```python
from build123d import *

# Parameters (mm, degrees)
SKETCH2_W          = 3.5
SKETCH2_H          = 3.5
CUT_EXTRUDE1_DEPTH = 8.1086


with BuildPart() as part:
    # Sketch1 → Revolve1 (revolve)
    with BuildSketch(Plane.XY):
        Polygon((1.957910998, 0), (0, 0), (0, -2.01497422), (0, -7.1086), (3.0734, -7.1086), (3.0734, -3), (60, -3), (60, 0), align=None)
    revolve(axis=Axis((0, 0, 0), (0, -1, 0)))

    # Sketch2 → Cut-Extrude1 (cut, through all)
    with BuildSketch(Plane(origin=(0, 0, 0), x_dir=(1, 0, 0), z_dir=(0, 1, 0))):
        with BuildLine():
            Line((2.37773001, -1.17), (-2.37773001, -1.17))
            ThreePointArc((-2.37773001, -1.17), (0, 2.65), (2.37773001, -1.17))
        make_face()
        with Locations((-42.92, 0)):
            Rectangle(SKETCH2_W, SKETCH2_H)
        with Locations((0, -42.92)):
            Rectangle(SKETCH2_W, SKETCH2_H)
        with Locations((0, 42.92)):
            Rectangle(SKETCH2_W, SKETCH2_H)
        with Locations((42.92, 0)):
            Rectangle(SKETCH2_W, SKETCH2_H)
    extrude(amount=-CUT_EXTRUDE1_DEPTH, mode=Mode.SUBTRACT)


solid = part.part
```
Verification items for the finished model (mm, model axes). A direction names the side the tool comes from. Give positions to 0.01 mm unless a question says otherwise; leave off trailing zeros. Order: outer loops, then holes, each group sorted by start corner. A loop starts at its lowest first (then second) coordinate and runs counter-clockwise, first axis right, second up. Notation, with made-up numbers: M 17,-6.5 L 52,-6.5 A15 cw 52,10.5 Z; hole C 11.5,26.5 d6. An arc over 180 degrees is marked long. Return JSON: item names as keys, results as strings. Group by question number.
1) Section check D-D on x = -14. Record the cut outline in (y, z), and give its area (3 significant figures).
2) Section check B-B on y = -4.75. Record the cut outline in (x, z).
3) Scan lines: line 1 (Z direction, x = 0, y = -2); line 2 (Z direction, x = 0, y = -5.25); line 3 (Y direction, x = -8, z = -42). Record each from-to range of solid material in increasing order.
4) Section check A-A on x = 0. Record the cut outline in (y, z), and give its area (3 significant figures).
5) Access from +Z, -Z, +X, -X, +Y, -Y to the whole of each face (thin tool, end or side, straight path). Record for faces 1 (the face through (2.931, -5.026, 0.923)), 2 (the face through (-1.75, -1, -43)), 3 (the face through (-1, 0, -12)).
6) Section check C-C on z = 9.5. Record the cut outline in (x, y).
7) Mould release check, pull along Z, two halves, no side actions. Record for faces 4 (the face through (0, -7.109, 1.4)), 5 (the face through (0, -1, 41.17)), 6 (the face through (-59.94, -1.48, 2.64)), 7 (the face through (-43, -1, -1.75)): pulls with the +Z half, pulls with the -Z half, needs draft (parallel to the pull), parting line crosses it, or undercut.
8) Go/stop test with flat-tipped pins: pin 1 Ø1.5 at (x, y) = (0.5, -2) entering from +Z; pin 2 Ø2 at (y, z) = (-1, 40.5) entering from +X; pin 3 Ø4 at (x, y) = (-33.5, -3) entering from +Z; pin 4 Ø3 at (x, y) = (-12, -6) entering from +Z. Record where each tip stops, or that it passes through.
Answer block:
{
 "1": {"outline": "M -3,-58.34 L 0,-58.34 L 0,58.34 L -3,58.34 Z", "area": "350 mm^2"},
 "2": {"outline": "C 0,0 d6.15; hole M -2.38,1.17 A2.65 ccw long 2.38,1.17 Z"},
 "3": {"line 1": "z = -60 to -44.67, -41.17 to -2.65, 1.17 to 41.17, 44.67 to 60", "line 2": "z = -3.07 to -2.65, 1.17 to 3.07", "line 3": "y = -3 to 0"},
 "4": {"outline": "M -7.11,-3.07 L -3,-3.07 L -3,-41.17 L 0,-41.17 L 0,-2.65 L -7.11,-2.65 Z; M -7.11,1.17 L 0,1.17 L 0,41.17 L -3,41.17 L -3,3.07 L -7.11,3.07 Z; M -3,-60 L 0,-60 L 0,-44.67 L -3,-44.67 Z; M -3,44.67 L 0,44.67 L 0,60 L -3,60 Z", "area": "337 mm^2"},
 "5": {"face 1": "-Y", "face 2": "+Y, -Y", "face 3": "+Z, -Z, +X, -X, +Y"},
 "6": {"outline": "M -59.24,-3 L 59.24,-3 L 59.24,0 L -59.24,0 Z"},
 "7": {"face 4": "needs draft", "face 5": "undercut", "face 6": "parting line crosses it", "face 7": "undercut"},
 "8": {"pin 1": "stops at z = 60", "pin 2": "stops at x = 45.16", "pin 3": "stops at z = 51.07", "pin 4": "passes through"}
}
